The figure shows three views and two pictorial views of one solid part (mm, origin at its lowest corner). Answer the questions. A direction names the side the tool comes from. Round coordinates to 2 decimals unless told otherwise and drop trailing zeros. Order: outer loops, then holes, each group sorted by start corner. A loop starts at its lowest first (then second) coordinate and runs counter-clockwise, first axis right, second up. Notation, with made-up numbers: M 89,-15 L 117,-15 A13 ccw 117,7 Z; hole C 4,-24 d1. An arc over 180 degrees is marked long. Answer as CSV lines item,"result".
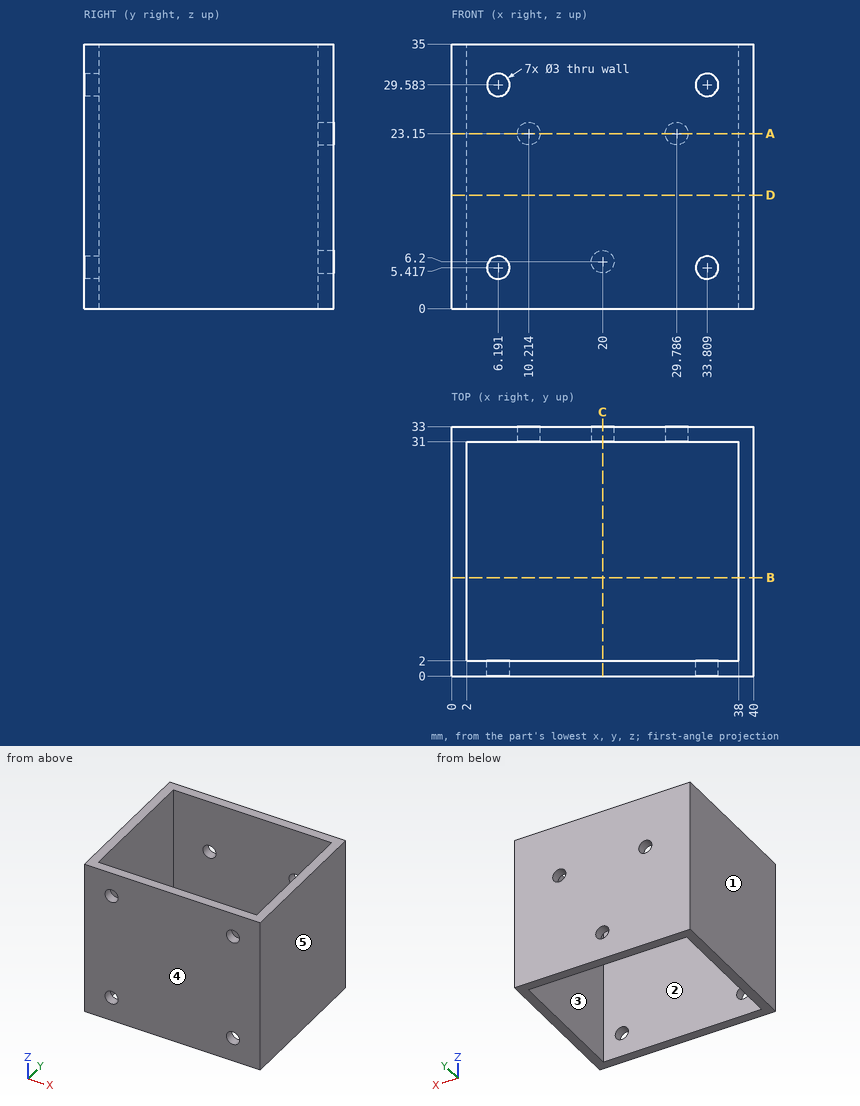
Item 1: A cutting plane is placed at D-D, the plane z = 15. Determine the outline of the cut face in (x, y).
Ans:
outline,"M 0,0 L 40,0 L 40,33 L 0,33 Z; hole M 2,2 L 38,2 L 38,31 L 2,31 Z"
Item 2: A cutting plane is placed at C-C, the plane x = 20. Determine the outline of the cut face in (y, z), and give its area (3 significant figures).
Ans:
outline,"M 0,0 L 2,0 L 2,35 L 0,35 Z; M 31,0 L 33,0 L 33,4.7 L 31,4.7 Z; M 31,7.7 L 33,7.7 L 33,35 L 31,35 Z"
area,"134 mm2"
Item 3: Find the intervals of material crossed by probe 1 along Y at (x, z) = (16, 14); probe 2 along X at (y, z) = (24, 26.5); probe 3 along Z at (x, y) = (20, 32), in increasing order. Write a range as [from, to].
Ans:
probe 1,"[0, 2], [31, 33]"
probe 2,"[0, 2], [38, 40]"
probe 3,"[0, 4.7], [7.7, 35]"
Item 4: A cutting plane is placed at A-A, the plane z = 23.15. Determine the outline of the cut face in (x, y), and give its area (3 significant figures).
Ans:
outline,"M 0,0 L 40,0 L 40,33 L 31.29,33 L 31.29,31 L 38,31 L 38,2 L 2,2 L 2,31 L 8.71,31 L 8.71,33 L 0,33 Z; M 11.71,31 L 28.29,31 L 28.29,33 L 11.71,33 Z"
area,"264 mm2"
Item 5: A tool of negligible diameter and unlimited length cuts with its end or side. For the marked faces 1 and 2, from which of +Z, -Z, +X, -X, +Y, -Y can it reach the whole face along a straight path? Write none if from no direction.
Ans:
face 1,"+Z, -Z, -X, +Y, -Y"
face 2,"+Z, -Z"
Item 6: Determine the mould class of the marked faces 3, 4 and 5 for opening direction X: +X half, -X half, draft (parallel to the pull), parting line (faces both ways), or undercut.
Ans:
face 3,"undercut"
face 4,"draft"
face 5,"+X half"
Item 7: Flat-ended cylindrical pins translate along their axes: pin 1 (5 mm diameter, centred on x = 34, y = 11.5, fed in from +Z); pin 2 (2.5 mm diameter, centred on x = 33.81, z = 5.42, fed in from -Y). Find the tip coordinate at first contact, or state that the pin passes through.
Ans:
pin 1,"through"
pin 2,"y = 31"
Item 8: A cutting plane is placed at B-B, the plane y = 13. Determine the outline of the cut face in (x, z), and give its area (3 significant figures).
Ans:
outline,"M 0,0 L 2,0 L 2,35 L 0,35 Z; M 38,0 L 40,0 L 40,35 L 38,35 Z"
area,"140 mm2"
